Part model, mm, in its own coordinate system. Face numbers are marked on the shaded views. A direction names the side the tool comes from. Give positions to 0.01 mm unless a question says otherwise; leave off trailing zeros. Write each loop counter-clockwise with the first axis right and the second up, starting at its lowest first coordinate (ties: lowest second). Pieces come first, ordered by that corner, then holes.
```python
from build123d import *

# Parameters (mm, degrees)
BASE_FLANGE2_DEPTH = 50
SKETCH14_R         = 1.7500000000000004
CUT_EXTRUDE1_DEPTH = 10
CUT_EXTRUDE2_DEPTH = 10
CHAMFER1_SIZE      = 40
CHAMFER1_SIZE2     = 10
FILLET1_R          = 1
CUT_EXTRUDE3_DEPTH = 10


# Sheet-metal steps are written as plain solids
with BuildPart() as part:
    # Sketch13 → Base-Flange2 (new body)
    with BuildSketch(Plane.XY):
        with BuildLine():
            Line((0, 0), (0, 150))
            ThreePointArc((0, 150), (17.155581462513624, 222.67220926874307), (64.99999999999997, 279.99999999999994))
            Line((64.99999999999997, 279.99999999999994), (67.99999999999997, 275.99999999999994))
            ThreePointArc((67.99999999999997, 275.99999999999994), (21.627717417513225, 220.4361412912433), (5, 150))
            Line((5, 150), (5, 0))
            Line((5, 0), (0, 0))
        make_face()
    extrude(amount=BASE_FLANGE2_DEPTH)

    # Sketch14 → Cut-Extrude1 (cut)
    with BuildSketch(Plane(origin=(5, 0, 0), x_dir=(0, 0, -1), z_dir=(1, 0, 0))):
        with Locations((-10.500030729924669, 141.8914274868206)):
            Circle(SKETCH14_R)
        with Locations((-10.500008780040803, 41.896427486823015)):
            Circle(SKETCH14_R)
    extrude(amount=-CUT_EXTRUDE1_DEPTH, mode=Mode.SUBTRACT)

    # Sketch15 → Cut-Extrude2 (cut)
    with BuildSketch(Plane.ZY):
        Polygon((0, 0), (20.000000000000004, 0), (19.999999999999996, 25), (0, 25), align=None)
        Polygon((6.94e-15, 80), (20.000000000000007, 80), (20.000000000000004, 100), (0, 100), align=None)
    extrude(amount=-CUT_EXTRUDE2_DEPTH, mode=Mode.SUBTRACT)

    # Chamfer1
    chamfer1_edges = [part.edges().sort_by_distance(p)[0] for p in [
        (66.49999999999997, 277.99999999999994, 50),
    ]]
    chamfer1_side = [part.faces().sort_by_distance(p)[0] for p in [
        (2.88138855415232, 75, 50),
    ]]
    chamfer(chamfer1_edges, length=CHAMFER1_SIZE, length2=CHAMFER1_SIZE2, reference=chamfer1_side[0])

    # Fillet1
    fillet1_edges = [part.edges().sort_by_distance(p)[0] for p in [
        (2.5, 0, 50),
        (2.5, 80, 6.94e-15),
        (2.5, 100, 0),
        (2.5, 25, 0),
        (2.5, 25, 19.999999999999996),
        (2.5, 0, 20.000000000000004),
        (2.5, 100, 20.000000000000004),
        (2.5, 80, 20.000000000000007),
        (66.49999999999997, 277.99999999999994, 0),
        (66.49999999999996, 277.99999999999994, 40),
        (37.54920679025358, 249.93439094632848, 50),
    ]]
    fillet(fillet1_edges, radius=FILLET1_R)

    # Sketch16 → Cut-Extrude3 (cut)
    with BuildSketch(Plane(origin=(5, 0, 0), x_dir=(0, 0, -1), z_dir=(1, 0, 0))):
        Polygon((-40, 140.1414274868206), (-40.00000000000002, 110.1414274868206), (-45.000000000000014, 110.1414274868206), (-45, 140.1414274868206), align=None)
    extrude(amount=-CUT_EXTRUDE3_DEPTH, mode=Mode.SUBTRACT)


solid = part.part
```
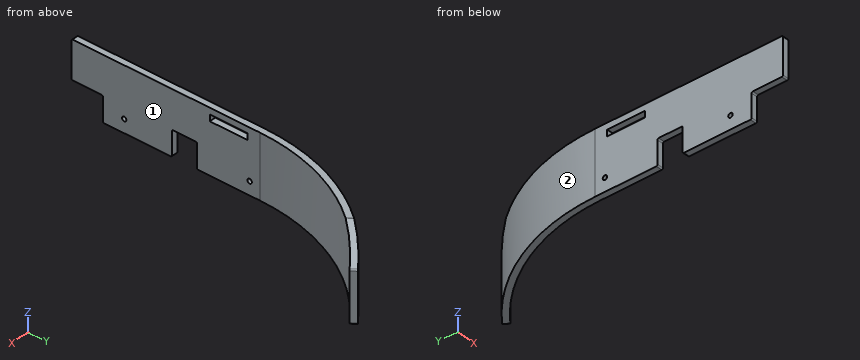
1) Saw through at C-C, the plane z = 30.5. Write the cut outline in (x, y).
Answers follow:
outline: (0, 0) - (5, 0) - (5, 150) arc R157.5 cw to (68, 276) - (65, 280) arc R162.5 ccw to (0, 150) - close
2) Saw through at A-A, the plane z = 5. Write the cut outline in (x, y), then the cut area to 3 significant figures.
Answers follow:
outline: (0, 25) - (5, 25) - (5, 80) - (0, 80) - close; (0, 100) - (5, 100) - (5, 150) arc R157.5 cw to (68, 276) - (65, 280) arc R162.5 ccw to (0, 150) - close
area: 1,270 mm2
3) 3-axis set-ups, long thin cutter, end or side, ignore diameter. For the marked faces 1 and 2: which of +Z, -Z, +X, -X, +Y, -Y reach the whole face in a straight line?
Answers follow:
face 1: +Z, -Z, +X, -Y
face 2: +Z, -Z, -X, +Y
4) Saw through at B-B, the plane y = 126. Write the cut outline in (x, z), then the cut area to 3 significant figures.
Answers follow:
outline: (0, 0) - (5, 0) - (5, 40) - (0, 40) - close; (0, 45) - (5, 45) - (5, 50) - (0, 50) - close
area: 225 mm2
5) Pin check, flat tips, straight feed: pin 1 Ø5.5 at (x, z) = (2, 11.5) entering from -Y; pin 2 Ø5.5 at (x, y) = (2.5, 88) entering from -Z; pin 3 Ø4 at (x, z) = (27, 28) entering from -Y; pin 4 Ø3 at (y, z) = (41.9, 10.5) entering from -X. Stop position of each tip, or through.
Answers follow:
pin 1: stops at y = 25
pin 2: stops at z = 20
pin 3: stops at y = 226.81
pin 4: passes through
6) Wall check: L1, parallel to Z at x = 4, y = 113; L2, parallel to Z at x = 4.5, y = 84; L3, parallel to X at y = 141, z = 28.5. Give the ranges that are in metal, low to high.
Answers follow:
L1: z = 0 to 40, 45 to 50
L2: z = 20 to 50
L3: x = 0 to 5
7) Saw through at D-D, the plane x = 44. Write the cut outline in (y, z), then the cut area to 3 significant figures.
Answers follow:
outline: (253.75, 0) - (261.19, 0) - (261.19, 47.02) - (253.75, 48.14) - close
area: 354 mm2
